Design review of the part built by this model. Coordinates are the model's own, in mm. A direction names the side the tool comes from. Give positions to 0.01 mm unless a question says otherwise; leave off trailing zeros. Order: outer loops, then holes, each group sorted by start corner. A loop starts at its lowest first (then second) coordinate and runs counter-clockwise, first axis right, second up. Notation, with made-up numbers: (76, 68.5) -> (112, 68.5) arc R29 cw to (112, 97.5) -> close; hole circle Ø6 at (62.5, 39). An arc over 180 degrees is marked (long way). One line per item, written item: value.
from build123d import *

# Parameters (mm, degrees)
SKETCH_1_R               = 1.55
SKETCH_1_W               = 14.9
SKETCH_1_H               = 10
EXTRUDE_1_DEPTH          = 2
FILLET_1_R               = 1
HOLE_WIZARD_1_AT_2_COUNT = 2
HOLE_WIZARD_1_AT_2_PITCH = 15
FILLET_2_R               = 3


with BuildPart() as part:
    # 草图1 → 凸台-拉伸1 (new body)
    with BuildSketch(Plane.XY):
        Polygon((9.5, -12.5), (-9.5, -12.5), (-9.5, 12.5), (9.5, 12.5), (9.5, 17.5), (18.4, 17.5), (18.4, 2.5), (18.4, -7.5), (22.730127019, -5), (18.4, -12.5), align=None)
        with Locations((14.5, 13.5)):
            Circle(SKETCH_1_R, mode=Mode.SUBTRACT)
        with Locations((14.5, 5.5)):
            Circle(SKETCH_1_R, mode=Mode.SUBTRACT)
        with Locations((-4.5, 7.5)):
            Circle(SKETCH_1_R, mode=Mode.SUBTRACT)
        with Locations(Location((-4.5, -7.5, 0), (0, 0, 180))):
            Circle(SKETCH_1_R, mode=Mode.SUBTRACT)
        with Locations((7.95, -3.5)):
            Rectangle(SKETCH_1_W, SKETCH_1_H, mode=Mode.SUBTRACT)
    extrude(amount=EXTRUDE_1_DEPTH)

    # 圆角1
    fillet_1_edges = [part.edges().sort_by_distance(p)[0] for p in [
        (-9.5, 12.5, 1),
        (9.5, 12.5, 1),
        (9.5, 17.5, 1),
        (18.4, 17.5, 1),
        (18.4, -7.5, 1),
        (18.4, -12.5, 1),
        (-9.5, -12.5, 1),
        (0.5, 1.5, 1),
        (0.5, -8.5, 1),
        (15.4, -8.5, 1),
        (15.4, 1.5, 1),
    ]]
    fillet(fillet_1_edges, radius=FILLET_1_R)

    # 草图2 → 打孔尺寸(%根据十字)槽沉头木螺钉的类型1 (revolve, cut)
    with BuildSketch(Plane(origin=(-4.5, 7.5, 0), x_dir=(0, 1, 0), z_dir=(1, 0, 0))):
        Polygon((0, 0), (0, 2), (1.55, 2), (1.55, 1.75), (3.3, 0), align=None)
    hole_wizard_1 = revolve(axis=Axis((-4.5, 7.5, -6.35), (0, 0, 1)), mode=Mode.SUBTRACT)

    # 打孔尺寸(%根据十字)槽沉头木螺钉的类型1 at 2: 打孔尺寸(%根据十字)槽沉头木螺钉的类型1 ×2
    with Locations(*[(0, -i * HOLE_WIZARD_1_AT_2_PITCH, 0) for i in range(1, HOLE_WIZARD_1_AT_2_COUNT)]):
        add(hole_wizard_1, mode=Mode.SUBTRACT)

    # 圆角2
    fillet_2_edges = [part.edges().sort_by_distance(p)[0] for p in [
        (22.730127019, -5, 1),
    ]]
    fillet(fillet_2_edges, radius=FILLET_2_R)


solid = part.part
Item 1: Add section B-B on y = 7.5. Give the boundary of the cut face in (x, z), plus the area to 3 significant figures.
Returned:
outline: (-9.5, 0) -> (-7.8, 0) -> (-6.05, 1.75) -> (-6.05, 2) -> (-9.5, 2) -> close; (-2.95, 1.75) -> (-1.2, 0) -> (18.4, 0) -> (18.4, 2) -> (-2.95, 2) -> close
area: 46.5 mm²
Item 2: Add section A-A on x = -4.5. Give the boundary of the cut face in (y, z), plus the area to 3 significant figures.
Returned:
outline: (-12.5, 0) -> (-10.8, 0) -> (-9.05, 1.75) -> (-9.05, 2) -> (-12.5, 2) -> close; (-5.95, 1.75) -> (-4.2, 0) -> (4.2, 0) -> (5.95, 1.75) -> (5.95, 2) -> (-5.95, 2) -> close; (9.05, 1.75) -> (10.8, 0) -> (12.5, 0) -> (12.5, 2) -> (9.05, 2) -> close
area: 31.5 mm²
Item 3: Add section D-D on z = 0.6. Count the separate pieces of the cut face and the enclosed holes in it, plus the area to 3 significant figures.
Returned:
separate pieces: 1
enclosed holes: 5
area: 539 mm²
Item 4: To check wall thickness, follow line 1 along Y through (x, z) = (-4.5, 1.85); line 2 along Y through (x, z) = (14.25, 1.05); line 3 along Y through (x, z) = (10.5, 1). State the ranges of each line that lie inside material, in increasing order. Write a range as from..to.
Returned:
line 1: -12.5..-9.05, -5.95..5.95, 9.05..12.5
line 2: -12.5..-8.5, 1.5..3.97, 7.03..11.97, 15.03..17.5
line 3: -12.5..-8.5, 1.5..17.5
Item 5: Draft analysis for pull direction Y (two halves, no side actions). For faces 6 (the cylindrical face through (13.36, 14.55, 0.99)), 7 (the cylindrical face through (18.115, 17.199, 1.014)), 8 (the flat face through (4, -12.5, 1)), state which applies: pulls with the +Y half, pulls with the -Y half, needs draft (parallel to the pull), parting line crosses it, or undercut.
Returned:
face 6: undercut
face 7: pulls with the +Y half
face 8: pulls with the -Y half
Item 6: Clearance check with flat-ended pins moving along their axes: P1, Ø0.6, axis at x = 9, z = 0.5, coming from the +Y side; P2, Ø1.9, axis at x = 14.5, y = 5.5, coming from the +Z side; P3, Ø0.6, axis at y = 14.5, z = 1, coming from the -X side; P4, Ø0.6, axis at x = 0, z = 0.5, coming from the +Y side. State where each tip first meets the part, or that it passes through.
Returned:
P1: y = 12.9
P2: through
P3: x = 9.5
P4: y = 12.5
Item 7: Machinability: for faces 1 (the flat face through (0.5, -4, 1)), 2 (the flat face through (18.4, 5, 1)), 3 (the conical face through (-2.88, 7.14, 1.64)), 4 (the flat face through (19.14, -11.22, 0.99)), 5 (the flat face through (9.5, 15, 1)), which of the approach directions +Z, -Z, +X, -X, +Y, -Y give a long, thin tool a straight path to every point of the face, cutting with its end or side? Answer none if there is none.
Returned:
face 1: +Z, -Z
face 2: +Z, -Z, +X, +Y
face 3: -Z
face 4: +Z, -Z, +X, -Y
face 5: +Z, -Z, -X, +Y
Item 8: Add section C-C on x = 11. Give the boundary of the cut face in (y, z).
Returned:
outline: (-12.5, 0) -> (-8.5, 0) -> (-8.5, 2) -> (-12.5, 2) -> close; (1.5, 0) -> (17.5, 0) -> (17.5, 2) -> (1.5, 2) -> close
